Geometry: final body of the model. Coordinates: model frame, mm. Face numbers are marked on the shaded views. A direction names the side the tool comes from. Give positions to 0.01 mm unless a question says otherwise; leave off trailing zeros. Write each loop counter-clockwise with the first axis right and the second up, starting at its lowest first coordinate (ties: lowest second). Pieces come first, ordered by that corner, then holes. Notation, with made-up numbers: (56, 71) - (86, 71) arc R33 cw to (86, 100) - close; hole circle Ø5 at (-11.75, 15.5). An arc over 180 degrees is marked (long way). Return JSON: item names as keys, results as strings.
from build123d import *

# Parameters (mm, degrees)
F0_R          = 55.632666
F1_DEPTH      = 25.4
F2_DEPTH      = 103.378
F4_DEPTH      = 6.35
F4_DEPTH_BACK = 6.35


with BuildPart() as f1:
    # F0 (on Top) → F1 (new body)
    with BuildSketch(Plane.XY):
        with BuildLine():
            Line((-139.827257, 69.913628), (-139.827257, -69.913628))
            Line((-139.827257, -69.913628), (69.913628, -69.913628))
            ThreePointArc((69.913628, -69.913628), (0, 0), (69.913628, 69.913628))
            Line((69.913628, 69.913628), (-139.827257, 69.913628))
        make_face()
        with BuildLine():
            ThreePointArc((69.913628, 69.913628), (0, 0), (69.913628, -69.913628))
            ThreePointArc((69.913628, -69.913628), (119.350029, -49.436401), (139.827257, 0))
            ThreePointArc((139.827257, 0), (119.350029, 49.436401), (69.913628, 69.913628))
        make_face()
        with Locations((69.913628, 0)):
            Circle(F0_R, mode=Mode.SUBTRACT)
    extrude(amount=F1_DEPTH)

    # F0 (on Top) → F2 (join)
    with BuildSketch(Plane.XY):
        with BuildLine():
            ThreePointArc((69.913628, 69.913628), (0, 0), (69.913628, -69.913628))
            ThreePointArc((69.913628, -69.913628), (119.350029, -49.436401), (139.827257, 0))
            ThreePointArc((139.827257, 0), (119.350029, 49.436401), (69.913628, 69.913628))
        make_face()
        with Locations((69.913628, 0)):
            Circle(F0_R, mode=Mode.SUBTRACT)
    extrude(amount=F2_DEPTH)

    # F3 (on Front) → F4 (join, two sides)
    with BuildSketch(Plane.XZ) as f4_sk:
        Polygon((14.280962, 83.201781), (-60.483344, 25.4), (14.280962, 25.4), align=None)
    extrude(amount=F4_DEPTH)
    extrude(f4_sk.sketch, amount=-F4_DEPTH_BACK)


solid = f1.part
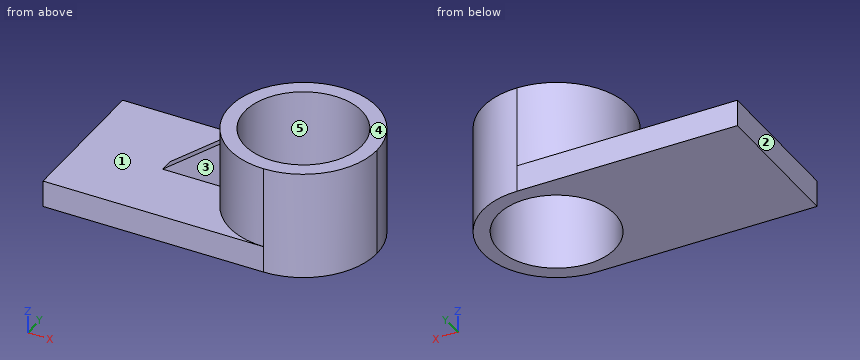
Q1. Section query A-A, the plane z = 57. Return the cut outline in (x, y).
Answer key:
{"outline": "(-19.61, -6.35) - (0.29, -6.35) arc R69.91 ccw to (69.91, -69.91) arc R69.91 ccw to (69.91, 69.91) arc R69.91 ccw to (0.29, 6.35) - (-19.61, 6.35) - close; hole circle Ø111.27 at (69.91, 0)"}
Q2. Set-up query: the marked faces 1 and 2. Return all of +Z, -Z, +X, -X, +Y, -Y with unobstructed straight access to the full face (end or side cutting, diameter ignored); none if empty.
Answer key:
{"face 1": "+Z, -X", "face 2": "+Z, -Z, -X, +Y, -Y"}
Q3. Section query D-D, the plane x = -56. Return the cut outline in (y, z).
Answer key:
{"outline": "(-69.91, 0) - (69.91, 0) - (69.91, 25.4) - (6.35, 25.4) - (6.35, 28.87) - (-6.35, 28.87) - (-6.35, 25.4) - (-69.91, 25.4) - close"}
Q4. Section query B-B, the plane x = 47.5. Return the cut outline in (y, z), plus the area to 3 significant figures.
Answer key:
{"outline": "(-69.91, 0) - (-50.92, 0) - (-50.92, 103.38) - (-66.22, 103.38) - (-66.22, 25.4) - (-69.91, 25.4) - close; (50.92, 0) - (69.91, 0) - (69.91, 25.4) - (66.22, 25.4) - (66.22, 103.38) - (50.92, 103.38) - close", "area": "3,350 mm^2"}
Q5. Material intervals for probe 1 along Z at (x, y) = (-89, -53); probe 2 along Y at (x, z) = (87, 59.5); probe 3 along X at (y, z) = (-15.5, 32), sorted ascending. Write a range as [from, to].
Answer key:
{"probe 1": "z = [0, 25.4]", "probe 2": "y = [-67.79, -52.94], [52.94, 67.79]", "probe 3": "x = [1.74, 16.48], [123.34, 138.09]"}
Q6. Mould query, pull axis Y, two halves, no side actions, for the marked faces 3, 4 and 5. Classes: pulls with the +Y half, pulls with the -Y half, needs draft (parallel to the pull), parting line crosses it, or undercut.
Answer key:
{"face 3": "pulls with the -Y half", "face 4": "needs draft", "face 5": "undercut"}
Q7. Section query C-C, the plane y = 17.5. Return the cut outline in (x, z).
Answer key:
{"outline": "(-139.83, 0) - (17.11, 0) - (17.11, 103.38) - (2.23, 103.38) - (2.23, 25.4) - (-139.83, 25.4) - close; (122.72, 0) - (137.6, 0) - (137.6, 103.38) - (122.72, 103.38) - close"}
Q8. Pin query (flat end, axial travel): P1, Ø2, axis at y = -7.5, z = 28.5, coming from the -X side; P2, Ø4, axis at y = -0.5, z = 65, coming from the -X side; P3, Ø2, axis at x = 22.5, z = 83.5, coming from the +Y side. Return the tip coordinate at first contact, or that it passes through.
Answer key:
{"P1": "stops at x = 0.3", "P2": "stops at x = -11.85", "P3": "stops at y = 52.28"}
